Read the model definition and answer for the solid it produces. Units are mm, in the model's axes. Give positions to 0.01 mm unless a question says otherwise; leave off trailing zeros. Loops run counter-clockwise (first coordinate to the right, second up) from the corner with the lowest first, then second, coordinate; pieces in that order, holes last. Notation, with made-up numbers: (-32, 88.5) -> (-16, 88.5) arc R25 cw to (-16, 124.5) -> close; hole circle Ø11 at (22.5, 70). An arc over 180 degrees is marked (long way). Write each question's results on one line, items separated by ' | '. Start each with the question number.
Item 1: Section B-B on x = 486 is taken. Write down the section's boundary in (y, z).
Item 2: Section C-C on y = 248 is taken. State how many separate pieces and enclosed holes the cut face has, and give its area (3 significant figures).
Item 3: Section A-A on z = 101 is taken. Write down the section's boundary in (x, y).
Item 4: Find the intervals of material crossed by line 1 (Z direction, x = -74.5, y = 375); line 2 (Z direction, x = -99.5, y = 259); line 3 (Z direction, x = -437.5, y = 290), in increasing order.
Item 5: Each of these flat-tipped pins is pushed along its axis until it touches: P1, Ø6, axis at x = -29.5, y = -49.5, coming from the -Z side; P2, Ø1.5, axis at x = 365, y = -395, coming from the +Z side; P3, Ø4, axis at y = -124.5, z = 120.5, coming from the +X side. Where does it stop, or does it pass through?
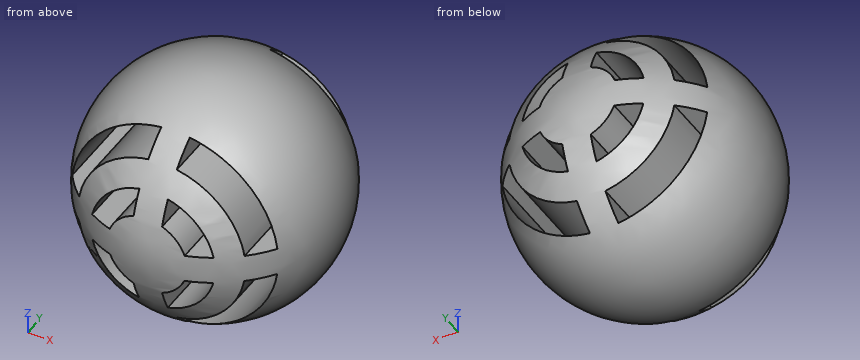
```python
from build123d import *

# Parameters (mm, degrees)
F3_DEPTH      = 635.001
F3_DEPTH_BACK = 635.001


with BuildPart() as f1:
    # F0 (on Front) → F1 (revolve)
    with BuildSketch(Plane.XZ):
        with BuildLine():
            Line((0, -635), (0, 635))
            ThreePointArc((0, 635), (-635, 0), (0, -635))
        make_face()
    revolve(axis=Axis((0, 0, 0), (0, 0, -1)))

    # F2 (on Front) → F3 (cut, two sides)
    with BuildSketch(Plane.XZ) as f3_sk:
        with BuildLine():
            Line((-68.7930285931, 419.6385528851), (-68.7930285931, 521.0308650177))
            ThreePointArc((-68.7930285931, 521.0308650177), (-371.924238815, 371.3192745683), (-521.1421629514, 67.9447501898))
            Line((-521.1421629514, 67.9447501898), (-419.7767344341, 67.9447501898))
            ThreePointArc((-419.7767344341, 67.9447501898), (-300.9937475259, 300.3860179849), (-68.7930285931, 419.6385528851))
        make_face()
        with BuildLine():
            ThreePointArc((521.1421629514, 67.9447501898), (374.4532709289, 368.7687499975), (75.908228755, 520.0419058993))
            Line((75.908228755, 520.0419058993), (75.908228755, 418.4100102265))
            ThreePointArc((75.908228755, 418.4100102265), (303.5331453171, 297.8197870263), (419.7767344341, 67.9447501898))
            Line((419.7767344341, 67.9447501898), (521.1421629514, 67.9447501898))
        make_face()
        with BuildLine():
            ThreePointArc((75.908228755, -520.0419058993), (372.1123300156, -371.1307814429), (520.2405848329, -74.5344012976))
            Line((520.2405848329, -74.5344012976), (418.6569226392, -74.5344012976))
            ThreePointArc((418.6569226392, -74.5344012976), (301.1831350648, -300.1961275617), (75.908228755, -418.4100102265))
            Line((75.908228755, -418.4100102265), (75.908228755, -520.0419058993))
        make_face()
        with BuildLine():
            Line((-68.7930285931, 189.9623297509), (-68.7930285931, 308.2805801706))
            ThreePointArc((-68.7930285931, 308.2805801706), (-223.6558098066, 223.0414213394), (-308.4686496469, 67.9447501898))
            Line((-308.4686496469, 67.9447501898), (-190.2673866669, 67.9447501898))
            ThreePointArc((-190.2673866669, 67.9447501898), (-143.1787243942, 142.5412936248), (-68.7930285931, 189.9623297509))
        make_face()
        with BuildLine():
            ThreePointArc((187.7838931607, -74.5344012976), (143.3827538067, -142.3360580394), (75.908228755, -187.2327650671))
            Line((75.908228755, -187.2327650671), (75.908228755, -306.6061605719))
            ThreePointArc((75.908228755, -306.6061605719), (223.8483767569, -222.8481570861), (306.943023893, -74.5344012976))
            Line((306.943023893, -74.5344012976), (187.7838931607, -74.5344012976))
        make_face()
        with BuildLine():
            ThreePointArc((308.4686496469, 67.9447501898), (226.2216023369, 220.4386162392), (75.908228755, 306.6061605719))
            Line((75.908228755, 306.6061605719), (75.908228755, 187.2327650671))
            ThreePointArc((75.908228755, 187.2327650671), (145.8415996369, 139.8155761092), (190.2673866669, 67.9447501898))
            Line((190.2673866669, 67.9447501898), (308.4686496469, 67.9447501898))
        make_face()
        with BuildLine():
            Line((-68.7930285931, -521.0308650177), (-68.7930285931, -419.6385528851))
            ThreePointArc((-68.7930285931, -419.6385528851), (-298.6236470875, -302.7423215388), (-418.6569226392, -74.5344012976))
            Line((-418.6569226392, -74.5344012976), (-520.2405848329, -74.5344012976))
            ThreePointArc((-520.2405848329, -74.5344012976), (-369.5672096724, -373.6652520894), (-68.7930285931, -521.0308650177))
        make_face()
        with BuildLine():
            Line((-187.7838931607, -74.5344012976), (-306.943023893, -74.5344012976))
            ThreePointArc((-306.943023893, -74.5344012976), (-221.2548628141, -225.4233407934), (-68.7930285931, -308.2805801706))
            Line((-68.7930285931, -308.2805801706), (-68.7930285931, -189.9623297509))
            ThreePointArc((-68.7930285931, -189.9623297509), (-140.6727793886, -145.0149531823), (-187.7838931607, -74.5344012976))
        make_face()
    extrude(amount=-F3_DEPTH, mode=Mode.SUBTRACT)
    extrude(f3_sk.sketch, amount=F3_DEPTH_BACK, mode=Mode.SUBTRACT)


solid = f1.part
```
Findings:
1) outline: (-403, 67.94) arc R408.69 ccw to (-401.84, -74.53) -> (401.84, -74.53) arc R408.69 ccw to (403, 67.94) -> close; (-356.4, -200.02) arc R408.69 ccw to (356.4, -200.02) -> close; (-356.4, 200.02) -> (356.4, 200.02) arc R408.69 ccw to start
2) separate pieces: 1 | enclosed holes: 8 | area: 713,000 mm2
3) outline: (-515.76, -356.4) -> (-515.76, 356.4) arc R626.92 ccw to start; (-413.07, -471.59) arc R626.92 ccw to (-299.28, -550.87) -> (-299.28, 550.87) arc R626.92 ccw to (-413.07, 471.59) -> close; (-174.98, -602) arc R626.92 ccw to (174.98, -602) -> (174.98, 602) arc R626.92 ccw to (-174.98, 602) -> close; (299.28, -550.87) arc R626.92 ccw to (413.07, -471.59) -> (413.07, 471.59) arc R626.92 ccw to (299.28, 550.87) -> close; (515.76, -356.4) arc R626.92 ccw to (515.76, 356.4) -> close
4) line 1: -418.66 to -306.95, -187.8 to 187.8, 306.95 to 418.66 | line 2: -571.18 to -516.05, -413.44 to -299.78, -175.83 to 175.83, 299.78 to 413.44, 516.05 to 571.18 | line 3: -357.38 to -291.2, -74.53 to 67.94, 291.2 to 357.38
5) P1: z = -632.65 | P2: z = 219.43 | P3: x = 611.47
